Source: CAD feature listing. Evaluate the final solid. Frame: model axes, mm. Give positions to 0.01 mm unless a question says otherwise; leave off trailing zeros. Order: outer loops, then holes, each group sorted by start corner. A loop starts at its lowest first (then second) coordinate and runs counter-clockwise, first axis right, second up. Notation, with made-up numbers: (-31.5, 34) - (-1.5, 34) arc R15 cw to (-1.5, 62) - close; hole circle Ø5 at (3, -13). An arc over 180 degrees is marked (long way). Answer as CSV lines item,"result".
```python
from build123d import *

# Parameters (mm, degrees)
YUGO_DEPTH          = 4
OJO_CABLE_PROFILE_R = 2


with BuildPart() as part:
    # Sk_Yugo → Yugo (new body)
    with BuildSketch(Plane(origin=(-318.901689809, 238.632958282, 0), x_dir=(0, 0, 1), z_dir=(-0.800654275017383, 0.5991266409502992, 0))):
        Polygon((-14, 203.763792808), (14, 203.763792808), (6, 220.763792808), (-6, 220.763792808), align=None)
    extrude(amount=YUGO_DEPTH)

    # Ojo_cable: sweep along a curve in space
    with BuildLine() as ojo_cable_path:
        Line((-190.029452392, 409.184726197, 0), (-194.833378042, 412.779486043, 0))
    # Ojo_cable profile (on start of the path) → Ojo_cable (sweep, cut)
    with BuildSketch(Plane(origin=(-190.029452392, 409.184726197, 0), x_dir=(-0.5991266409502979, -0.8006542750173841, 0), z_dir=(-0.8006542750173841, 0.5991266409502979, 0))):
        Circle(OJO_CABLE_PROFILE_R)
    sweep(path=ojo_cable_path.line, mode=Mode.SUBTRACT)


solid = part.part
```
(1) Cut plane B-B (x = -187.75). Return loops of the section in (y, z), then the cut area to 3 significant figures.
Completed:
outline,"(413.9, -6.87) - (416.22, -6) - (416.22, 6) - (413.9, 6.87) - close"
area,"29.9 mm²"
(2) Cut plane A-A (z = 5.5). Return loops of the section in (x, y).
Completed:
outline,"(-200.02, 404.17) - (-196.82, 401.78) - (-186.64, 415.39) - (-189.84, 417.78) - close"
(3) Mould query, pull axis Y, two halves, no side actions, for faces 1 (the flat face through (-192.789, 407.166, -0.196)), 2 (the flat face through (-188.215, 416.57, 0.084)), 3 (the cylindrical face through (-191.26, 412.6, 0.09)). Classes: released by +Y, released by -Y, zero draft, split by the parting line, or undercut.
Completed:
face 1,"released by -Y"
face 2,"released by +Y"
face 3,"undercut"
(4) Ray query, line 1 (Z direction, x = -192, y = 412.75); line 2 (Y direction, x = -198.5, z = 6.5); line 3 (Y direction, x = -193.5, z = -7). Return the intervals inside material, ascending. Write a range as from..to.
Completed:
line 1,"-8.51..-1.09, 1.09..8.51"
line 2,"403.03..406.21"
line 3,"406.22..412.89"
(5) Contact query for flat-ended pins moving along their axis: pin 1 (2 mm diameter, centred on y = 408, z = 5.5, fed in from -X); pin 2 (3 mm diameter, centred on x = -198.5, z = -9.5, fed in from -Y); pin 3 (8 mm diameter, centred on x = -198.5, y = 409, fed in from +Z); pin 4 (2 mm diameter, centred on x = -189.5, y = 409, fed in from -Z). Output: stop coordinate, or through.
Completed:
pin 1,"x = -197.91"
pin 2,"y = 401.91"
pin 3,"z = 13.46"
pin 4,"through"
